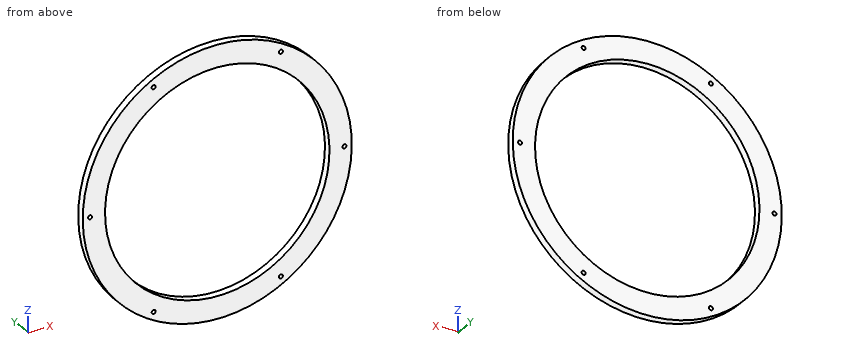
from build123d import *

# Parameters (mm, degrees)
SKETCH_1_R               = 175
SKETCH_1_R_2             = 146
EXTRUDE_1_DEPTH          = 10
SKETCH_2_R               = 2.6
CUT_EXTRUDE_1_DEPTH      = 248.68932153
PATTERN_CIRCULAR_1_COUNT = 6


with BuildPart() as part:
    # Эскиз1 → Бобышка-Вытянуть1 (new body)
    with BuildSketch(Plane(origin=(0, 0, 0), x_dir=(1, 0, 0), z_dir=(0, 1, 0))):
        with Locations(Location((0, 0, 0), (0, 0, 270))):
            Circle(SKETCH_1_R)
        with Locations(Location((0, 0, 0), (0, 0, 270))):
            Circle(SKETCH_1_R_2, mode=Mode.SUBTRACT)
    extrude(amount=EXTRUDE_1_DEPTH)

    # Эскиз2 → Вырез-Вытянуть1 (cut, through all)
    with BuildSketch(Plane(origin=(0, 10, 0), x_dir=(1, 0, 0), z_dir=(0, 1, 0))):
        with Locations(Location((-165.5, 0, 0), (0, 0, 270))):
            Circle(SKETCH_2_R)
    cut_extrude_1 = extrude(amount=-CUT_EXTRUDE_1_DEPTH, mode=Mode.SUBTRACT)

    # Круговой массив1: Вырез-Вытянуть1 ×6 about axis
    pattern_circular_1_axis = Axis((0, 0, 0), (0, 1, 0))
    for i in range(1, PATTERN_CIRCULAR_1_COUNT):
        add(cut_extrude_1.rotate(pattern_circular_1_axis, i * 360 / PATTERN_CIRCULAR_1_COUNT), mode=Mode.SUBTRACT)


solid = part.part
Design review of the part built by this model. Coordinates are the model's own, in mm. Give positions to 0.01 mm unless a question says otherwise; leave off trailing zeros. Loops run counter-clockwise (first coordinate to the right, second up) from the corner with the lowest first, then second, coordinate; pieces in that order, holes last. Notation, with made-up numbers: (80.25, 73) - (94.25, 73) arc R16 ccw to (94.25, 93) - close; hole circle Ø11 at (-13, 45.25). An arc over 180 degrees is marked (long way). Write item = value, one per line.
1) Clearance check with flat-ended pins moving along their axes: pin 1 Ø7 at (x, z) = (82.75, -143.33) entering from -Y; pin 2 Ø3 at (y, z) = (7, -129.5) entering from +X; pin 3 Ø6 at (y, z) = (6.5, 46.5) entering from -X; pin 4 Ø2 at (x, y) = (-91.5, 3) entering from -Z. State where each tip first meets the part, or that it passes through.
Result sheet:
pin_1 = 0
pin_2 = 119.34
pin_3 = -169.51
pin_4 = -149.78
2) Take a section at C-C on y = 3. State the section outline as (x, z) points.
Result sheet:
outline = circle Ø350 at (0, 0); hole circle Ø5.2 at (-165.5, 0); hole circle Ø292 at (0, 0); hole circle Ø5.2 at (-82.75, -143.33); hole circle Ø5.2 at (-82.75, 143.33); hole circle Ø5.2 at (82.75, -143.33); hole circle Ø5.2 at (82.75, 143.33); hole circle Ø5.2 at (165.5, 0)
3) Take a section at B-B on z = 109. State the section outline as (x, y) points.
Result sheet:
outline = (-136.91, 0) - (-97.13, 0) - (-97.13, 10) - (-136.91, 10) - close; (97.13, 0) - (136.91, 0) - (136.91, 10) - (97.13, 10) - close
4) To check wall thickness, follow line 1 (Z direction, x = -82.75, y = 8); line 2 (X direction, y = 6.5, z = 130.5); line 3 (Z direction, x = -37.5, y = 8). State the ranges of each line that lie inside material, in increasing order.
Result sheet:
line_1 = -154.2 to -145.93, -140.73 to -120.28, 120.28 to 140.73, 145.93 to 154.2
line_2 = -116.6 to -65.47, 65.47 to 116.6
line_3 = -170.93 to -141.1, 141.1 to 170.93
5) Take a section at A-A on x = 0. State the section outline as (y, z) points.
Result sheet:
outline = (0, -175) - (10, -175) - (10, -146) - (0, -146) - close; (0, 146) - (10, 146) - (10, 175) - (0, 175) - close
